from build123d import *

# Parameters (mm, degrees)
SKETCH1_W                = 69.85
SKETCH1_H                = 76.2
BOSS_EXTRUDE1_DEPTH      = 6.35
M5_CLEARANCE_HOLE1_D     = 5.3
M5_CLEARANCE_HOLE1_DEPTH = 6.35
M5_CLEARANCE_HOLE1_TIP   = 1.59228064
CUT_EXTRUDE1_DEPTH       = 104.565365832
CUT_EXTRUDE2_DEPTH       = 104.565365832


with BuildPart() as part:
    # Sketch1 → Boss-Extrude1 (new body)
    with BuildSketch(Plane.XY):
        with Locations((34.925, 38.1)):
            Rectangle(SKETCH1_W, SKETCH1_H)
    extrude(amount=BOSS_EXTRUDE1_DEPTH)

    # M5 Clearance Hole1
    with Locations(Plane(origin=(6.35, 68.1, 6.35), x_dir=(1, 0, 0), z_dir=(0, 0, 1))):
        with Locations((0, 0), (0, -60)):
            Hole(M5_CLEARANCE_HOLE1_D / 2, depth=M5_CLEARANCE_HOLE1_DEPTH)
            with Locations((0, 0, -(M5_CLEARANCE_HOLE1_DEPTH + M5_CLEARANCE_HOLE1_TIP / 2))):  # 118° drill point
                Cone(0, M5_CLEARANCE_HOLE1_D / 2, M5_CLEARANCE_HOLE1_TIP, mode=Mode.SUBTRACT)

    # Sketch4 → Cut-Extrude1 (cut, through all)
    with BuildSketch(Plane.XY.offset(6.35)):
        with BuildLine():
            Line((64.77, 67.071875), (62.23, 67.071875))
            ThreePointArc((62.23, 67.071875), (59.451875, 69.85), (62.23, 72.628125))
            Line((62.23, 72.628125), (64.77, 72.628125))
            ThreePointArc((64.77, 72.628125), (67.548125, 69.85), (64.77, 67.071875))
        make_face()
        with BuildLine():
            Line((64.77, 9.128125), (62.23, 9.128125))
            ThreePointArc((62.23, 9.128125), (59.451875, 6.35), (62.23, 3.571875))
            Line((62.23, 3.571875), (64.77, 3.571875))
            ThreePointArc((64.77, 3.571875), (67.548125, 6.35), (64.77, 9.128125))
        make_face()
    extrude(amount=-CUT_EXTRUDE1_DEPTH, mode=Mode.SUBTRACT)

    # Sketch5 → Cut-Extrude2 (cut, through all)
    with BuildSketch(Plane.XY.offset(6.35)):
        with BuildLine():
            Line((66.9925, 17.78), (66.9925, 58.42))
            ThreePointArc((66.9925, 58.42), (62.23, 63.1825), (57.4675, 58.42))
            Line((57.4675, 58.42), (57.4675, 17.78))
            ThreePointArc((57.4675, 17.78), (62.23, 13.0175), (66.9925, 17.78))
        make_face()
        with BuildLine():
            ThreePointArc((66.9925, 17.78), (65.597596045, 14.412403955), (62.23, 13.0175))
            Line((62.23, 13.0175), (69.85, 13.0175))
            Line((69.85, 13.0175), (69.85, 63.1825))
            Line((69.85, 63.1825), (62.23, 63.1825))
            ThreePointArc((62.23, 63.1825), (65.597596045, 61.787596045), (66.9925, 58.42))
            Line((66.9925, 58.42), (66.9925, 17.78))
        make_face()
    extrude(amount=-CUT_EXTRUDE2_DEPTH, mode=Mode.SUBTRACT)


solid = part.part
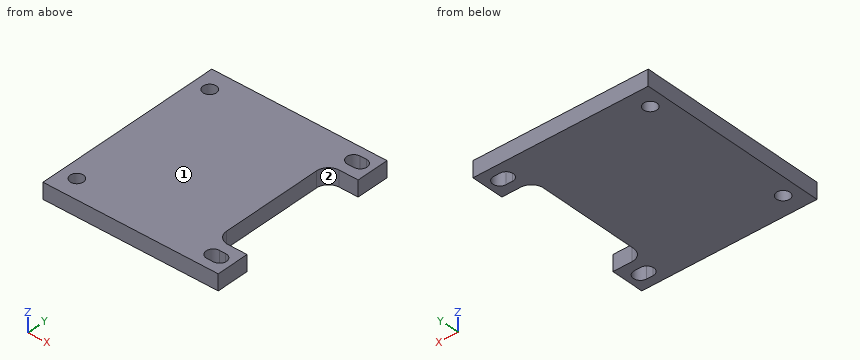
Design review of the part built by this model. Coordinates are the model's own, in mm. Face numbers are marked on the shaded views. Give positions to 0.01 mm unless a question says otherwise; leave off trailing zeros. Order: outer loops, then holes, each group sorted by start corner. A loop starts at its lowest first (then second) coordinate and runs counter-clockwise, first axis right, second up.
1. Add section C-C, the plane y = 8.1. State the section outline as (x, z) points.
Solution:
outline: (0, 0) - (3.7, 0) - (3.7, 6.35) - (0, 6.35) - close; (9, 0) - (60.07, 0) - (60.07, 6.35) - (9, 6.35) - close; (66.93, 0) - (69.85, 0) - (69.85, 6.35) - (66.93, 6.35) - close
2. Mouldability with a two-part tool opening along Y and no side actions: class the marked faces 1 and 2 as +Y half, -Y half, draft (parallel to the pull), parting line (faces both ways), or undercut.
Solution:
face 1: draft
face 2: undercut
3. Add section A-A, the plane z = 3.5. State how many separate pieces and enclosed holes the cut face has, then the cut area to 3 significant figures.
Solution:
separate pieces: 1
enclosed holes: 4
area: 4,590 mm2
4. For pin 1 Ø1.5 at (y, z) = (52.5, 1.5) entering from +X, flat-tipped, find the tip position at first contact; note if it passes through.
Solution:
pin 1: stops at x = 57.47
5. Add section D-D, the plane y = 33. State the section outline as (x, z) points.
Solution:
outline: (0, 0) - (57.47, 0) - (57.47, 6.35) - (0, 6.35) - close
6. To check wall thickness, follow L1, parallel to Y at x = 6.35, z = 2; L2, parallel to Y at x = 60.5, z = 0.5; L3, parallel to X at y = 68.1, z = 3.5. State the ranges of each line that lie inside material, in increasing order.
Solution:
L1: y = 0 to 5.45, 10.75 to 65.45, 70.75 to 76.2
L2: y = 0 to 4.18, 8.52 to 13.34, 62.86 to 67.68, 72.02 to 76.2
L3: x = 0 to 3.7, 9 to 60.07, 66.93 to 69.85
7. Add section B-B, the plane x = 6.35. State the section outline as (y, z) points.
Solution:
outline: (0, 0) - (5.45, 0) - (5.45, 6.35) - (0, 6.35) - close; (10.75, 0) - (65.45, 0) - (65.45, 6.35) - (10.75, 6.35) - close; (70.75, 0) - (76.2, 0) - (76.2, 6.35) - (70.75, 6.35) - close
